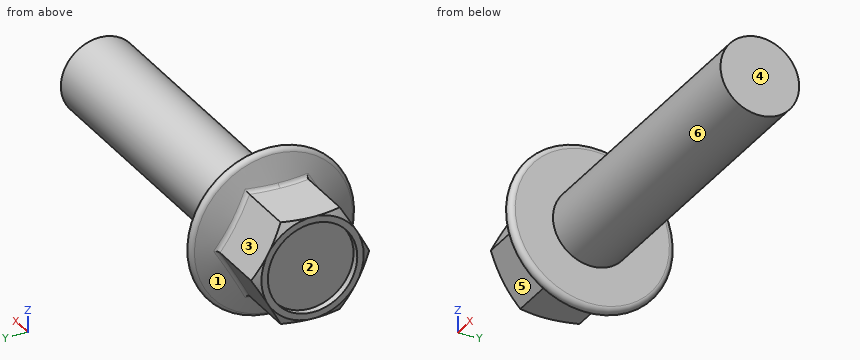
```python
from build123d import *

# Parameters (mm, degrees)
HEX_DIE_START     = -1e-06
SKETCH2_R         = 7.580831409
HEX_DIE_DEPTH     = 10.700001
FLANGEHEXFILLET_R = 0.6
SKETCH4_R         = 5.6875
INDENT_DEPTH      = 0.891666667


with BuildPart() as part:
    # BodySke → Base-Revolve (revolve)
    with BuildSketch(Plane.XY, mode=Mode.PRIVATE) as base_revolve_sk:
        Polygon((10.7, 5), (10.7, 7.505773672), (0.5806837, 7.505773672), (0, 6.5), (0, 0), (50.7, 0), (50.7, 5), align=None)
    revolve(base_revolve_sk.sketch.rotate(Axis((-25.4, 0, 0), (1, 0, 0)), 90), axis=Axis((-25.4, 0, 0), (1, 0, 0)))

    # Sketch2 → Hex-Die (cut)
    with BuildSketch(Plane(origin=(0, 0, 0), x_dir=(0, 0, -1), z_dir=(1, 0, 0)).offset(HEX_DIE_START)):
        Circle(SKETCH2_R)
        Polygon((-6.5, 3.752776766), (0, 7.505553532), (6.5, 3.752776766), (6.5, -3.752776766), (0, -7.505553532), (-6.5, -3.752776766), align=None, mode=Mode.SUBTRACT)
    extrude(amount=HEX_DIE_DEPTH, mode=Mode.SUBTRACT)

    # Sketch5 → Flange (revolve)
    with BuildSketch(Plane.XY, mode=Mode.PRIVATE) as flange_sk:
        with BuildLine():
            Line((5.688167263, 0), (9.342215165, 10.0394141))
            ThreePointArc((9.342215165, 10.0394141), (10.121553724, 10.489365427), (10.7, 9.8))
            Line((10.7, 9.8), (10.7, 0))
            Line((10.7, 0), (5.688167263, 0))
        make_face()
    revolve(flange_sk.sketch.rotate(Axis((0, 0, 0), (1, 0, 0)), 90), axis=Axis((0, 0, 0), (1, 0, 0)))

    # FlangeHexFillet
    flangehexfillet_edges = [part.edges().sort_by_distance(p)[0] for p in [
        (8.151404722, 1.884573799, 6.5),
        (8.053973794, 5.629165149, 3.25),
        (8.053973794, 5.629165149, -3.25),
        (8.053973786, 0, -6.5),
        (8.053973794, -5.629165149, -3.25),
        (8.053973794, -5.629165149, 3.25),
        (8.151404722, -1.884573799, 6.5),
    ]]
    fillet(flangehexfillet_edges, radius=FLANGEHEXFILLET_R)

    # Sketch4 → Indent (cut)
    with BuildSketch(Plane(origin=(0, 0, 0), x_dir=(0, 0, -1), z_dir=(1, 0, 0))):
        Circle(SKETCH4_R)
    extrude(amount=INDENT_DEPTH, mode=Mode.SUBTRACT)


solid = part.part
```
Source: CAD feature listing. Evaluate the final solid. Frame: model axes, mm. Face numbers are marked on the shaded views. A direction names the side the tool comes from. Round coordinates to 2 decimals unless told otherwise and drop trailing zeros. Loops run counter-clockwise (first coordinate to the right, second up) from the corner with the lowest first, then second, coordinate; pieces in that order, holes last. Notation, with made-up numbers: M 78,-15 L 97,-15 A25 cw 97,12 Z; hole C 35.5,87.25 d10. An arc over 180 degrees is marked long. Use a Markdown table: item, result. Add a question column.
1. Reachability of the marked faces 5 and 6 from +Z, -Z, +X, -X, +Y, -Y: full face, straight path, thin tool, end or side. Return the list, or none.
2. Line query: line 1 (Y direction, x = 0.6, z = 0); line 2 (Y direction, x = 26.5, z = 3); line 3 (X direction, y = 0.75, z = 5). Output: solid intervals per line, ascending.
3. Mould query, pull axis Z, two halves, no side actions, for the marked faces 1, 2, 3 and 4. Classes: pulls with the +Z half, pulls with the -Z half, needs draft (parallel to the pull), parting line crosses it, or undercut.
4. Contact query for flat-ended pins moving along their axis: P1, Ø8, axis at x = 40.5, y = -4.5, coming from the +Z side; P2, Ø5, axis at x = 10, y = -8, coming from the +Z side; P3, Ø6, axis at x = 10.5, y = 4.5, coming from the +Z side. Output: stop coordinate, or through.
5. Section query A-A on x = 35.5. Return the cut outline in (y, z), then the cut area to 3 significant figures.
Reported:
| question | item | result |
|---|---|---|
| 1 | face 5 | -Z, -X, -Y |
| 1 | face 6 | +X |
| 2 | line 1 | y = -7.51 to -5.69, 5.69 to 7.51 |
| 2 | line 2 | y = -4 to 4 |
| 2 | line 3 | x = 0.89 to 10.7 |
| 3 | face 1 | parting line crosses it |
| 3 | face 2 | undercut |
| 3 | face 3 | pulls with the +Z half |
| 3 | face 4 | needs draft |
| 4 | P1 | stops at z = 4.97 |
| 4 | P2 | stops at z = 8.94 |
| 4 | P3 | stops at z = 10.39 |
| 5 | outline | C 0,0 d10 |
| 5 | area | 78.5 mm² |
